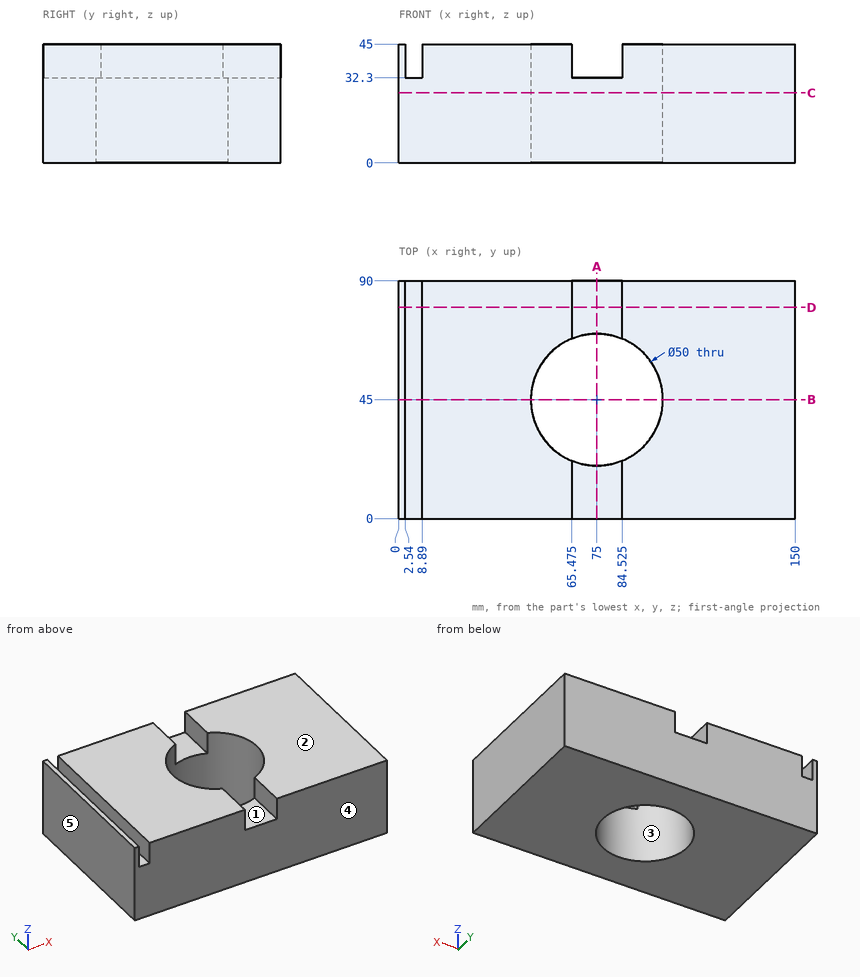
The drawing under review shows one solid part. Ordinate dimensions are in mm from its lowest x, y, z. A direction names the side the tool comes from. Round coordinates to 2 decimals unless told otherwise and drop trailing zeros. Write each loop counter-clockwise with the first axis right and the second up, starting at its lowest first coordinate (ties: lowest second). Pieces come first, ordered by that corner, then holes. Notation, with made-up numbers: (20.25, -5.5) - (65.25, -5.5) arc R8 cw to (65.25, -1.5) - close; hole circle Ø1 at (-18.75, 3). An arc over 180 degrees is marked (long way). Use a Markdown table: item, result. Add a question column.
1. Clearance check with flat-ended pins moving along their axes: pin 1 (5 mm diameter, centred on x = 37, z = 7.5, fed in from -Y); pin 2 (5 mm diameter, centred on x = 5.5, y = 25.5, fed in from +Z). State where each tip first meets the part, or that it passes through.
2. Mouldability with a two-part tool opening along X and no side actions: class the marked faces 3, 4 and 5 as +X half, -X half, draft (parallel to the pull), parting line (faces both ways), or undercut.
3. We need section B-B (y = 45). State the section outline as (x, z) points.
4. We need section C-C (z = 26.5). State the section outline as (x, y) points, then the cut area to 3 significant figures.
5. For the marked faces 1 and 2, list the 3-axis set-ups (+Z, -Z, +X, -X, +Y, -Y) from which the entire face can be reached by the end or side of a thin tool; tool diameter is ignored.
6. We need section D-D (y = 80). State the section outline as (x, z) points (3 decimals).
7. We need section A-A (x = 75). State the section outline as (y, z) points, then the cut area to 3 significant figures.
8. Wall thickness on probe 1 along X at (y, z) = (45, 25); probe 2 along X at (y, z) = (45, 36); probe 3 along Y at (x, z) = (75, 18): over which ranges is each line inside the solid? List them lowest first.
Output:
| question | item | result |
|---|---|---|
| 1 | pin 1 | stops at y = 0 |
| 1 | pin 2 | stops at z = 32.3 |
| 2 | face 3 | undercut |
| 2 | face 4 | draft |
| 2 | face 5 | -X half |
| 3 | outline | (0, 0) - (50, 0) - (50, 45) - (8.89, 45) - (8.89, 32.3) - (2.54, 32.3) - (2.54, 45) - (0, 45) - close; (100, 0) - (150, 0) - (150, 45) - (100, 45) - close |
| 4 | outline | (0, 0) - (150, 0) - (150, 90) - (0, 90) - close; hole circle Ø50 at (75, 45) |
| 4 | area | 11,500 mm2 |
| 5 | face 1 | +Z, +Y, -Y |
| 5 | face 2 | +Z, +X, -X, +Y, -Y |
| 6 | outline | (0, 0) - (150, 0) - (150, 45) - (84.525, 45) - (84.525, 32.3) - (65.475, 32.3) - (65.475, 45) - (8.89, 45) - (8.89, 32.3) - (2.54, 32.3) - (2.54, 45) - (0, 45) - close |
| 7 | outline | (0, 0) - (20, 0) - (20, 32.3) - (0, 32.3) - close; (70, 0) - (90, 0) - (90, 32.3) - (70, 32.3) - close |
| 7 | area | 1,290 mm2 |
| 8 | probe 1 | x = 0 to 50, 100 to 150 |
| 8 | probe 2 | x = 0 to 2.54, 8.89 to 50, 100 to 150 |
| 8 | probe 3 | y = 0 to 20, 70 to 90 |
